Check sheet for the modelled part. Datum: model origin and axes. Units: mm. Give positions to 0.01 mm unless a question says otherwise; leave off trailing zeros. Write each question's results on one line, items separated by ' | '. Start each with the question number.
1. Gauge pin test, flat ends, axial feed: pin 1 Ø1 at (x, z) = (6089.5, 1.5) entering from +Y; pin 2 Ø1 at (x, z) = (5918, 1.5) entering from +Y; pin 3 Ø2.5 at (x, y) = (6089.42, 2707.79) entering from -Z; pin 4 Ø1 at (y, z) = (2714.5, 1.5) entering from -X. Record the tip position at first contact, or that the pin passes through.
2. Material ranges on L1, parallel to X at y = 2715, z = 0.1; L2, parallel to X at y = 2711.75, z = 0.45, recorded low to high. Write a range as from..to.
3. Cross-section at A-A on z = 1.4. Count the separate pieces of the cut face and the enclosed holes in it, and give its area (3 significant figures).
from build123d import *

# Parameters (mm, degrees)
SKETCH1_R           = 1.4224
BOSS_EXTRUDE1_DEPTH = 3.175


with BuildPart() as part:
    # Sketch1 → Boss-Extrude1 (new body)
    with BuildSketch(Plane.XY):
        Polygon((6235.604848961, 2712.383832202), (6235.604848961, 2715.558832202), (6200.459551877, 2715.558832202), (6200.459551877, 2712.383832202), (6197.055951877, 2712.383832202), (6197.055951877, 2715.558832202), (6155.893298961, 2715.558832202), (6155.893298961, 2712.383832202), (6152.489698961, 2712.383832202), (6152.489698961, 2715.558832202), (6091.008998961, 2715.558832202), (6091.008998961, 2712.383832202), (6087.605398961, 2712.383832202), (6087.605398961, 2715.558832202), (6022.949698961, 2715.558832202), (6022.949698961, 2712.383832202), (6019.546098961, 2712.383832202), (6019.546098961, 2715.558832202), (5958.065398961, 2715.558832202), (5958.065398961, 2712.383832202), (5954.661798961, 2712.383832202), (5954.661798961, 2715.558832202), (5935.033948961, 2715.558832202), (5935.033948961, 2709.373932202), (5909.633948961, 2709.373932202), (5909.633948961, 2703.189032202), (6242.412048961, 2703.189032202), (6242.412048961, 2712.383832202), align=None)
        with Locations((5956.477898961, 2707.786432202)):
            Circle(SKETCH1_R, mode=Mode.SUBTRACT)
        with Locations((6021.362198961, 2707.786432202)):
            Circle(SKETCH1_R, mode=Mode.SUBTRACT)
        with Locations((6089.421498961, 2707.786432202)):
            Circle(SKETCH1_R, mode=Mode.SUBTRACT)
        with Locations((6154.305798961, 2707.786432202)):
            Circle(SKETCH1_R, mode=Mode.SUBTRACT)
        with Locations((6198.872051877, 2707.786432202)):
            Circle(SKETCH1_R, mode=Mode.SUBTRACT)
        with Locations((6237.420948961, 2707.786432202)):
            Circle(SKETCH1_R, mode=Mode.SUBTRACT)
    extrude(amount=BOSS_EXTRUDE1_DEPTH)


solid = part.part
Geometry says:
1) pin 1: y = 2712.38 | pin 2: y = 2709.37 | pin 3: through | pin 4: x = 5935.03
2) L1: 5935.03..5954.66, 5958.07..6019.55, 6022.95..6087.61, 6091.01..6152.49, 6155.89..6197.06, 6200.46..6235.6 | L2: 5935.03..6242.41
3) separate pieces: 1 | enclosed holes: 6 | area: 3,850 mm^2
